```python
from build123d import *

# Parameters (mm, degrees)
F1_DEPTH = 50.8
F2_R     = 2.975
F3_DEPTH = 12
F4_R     = 0.25
F5_DEPTH = 17


with BuildPart() as f1:
    # F0 (on Top) → F1 (new body)
    with BuildSketch(Plane.XY):
        Polygon((-1.9875, 6.35), (-6.35, 6.35), (-6.35, 1.9875), (-2.975, 1.9875), (-2.975, -1.9875), (-6.35, -1.9875), (-6.35, -6.35), (-1.9875, -6.35), (-1.9875, -2.975), (1.9875, -2.975), (1.9875, -6.35), (6.35, -6.35), (6.35, -1.9875), (2.975, -1.9875), (2.975, 1.9875), (6.35, 1.9875), (6.35, 6.35), (1.9875, 6.35), (1.9875, 2.975), (-1.9875, 2.975), align=None)
    extrude(amount=F1_DEPTH)

    # F2 (on face) → F3 (join)
    with BuildSketch(Plane.XY.offset(50.8)):
        Circle(F2_R)
    extrude(amount=F3_DEPTH)

    # F4 (on face) → F5 (cut)
    with BuildSketch(Plane.XY.offset(62.8)):
        with Locations((0, 1.5)):
            Circle(F4_R)
        with Locations((-1.426585, 0.463525)):
            Circle(F4_R)
        with Locations((-0.881678, -1.213525)):
            Circle(F4_R)
        with Locations((0.881678, -1.213525)):
            Circle(F4_R)
        Circle(F4_R)
        with Locations((1.426585, 0.463525)):
            Circle(F4_R)
    extrude(amount=-F5_DEPTH, mode=Mode.SUBTRACT)


solid = f1.part
```
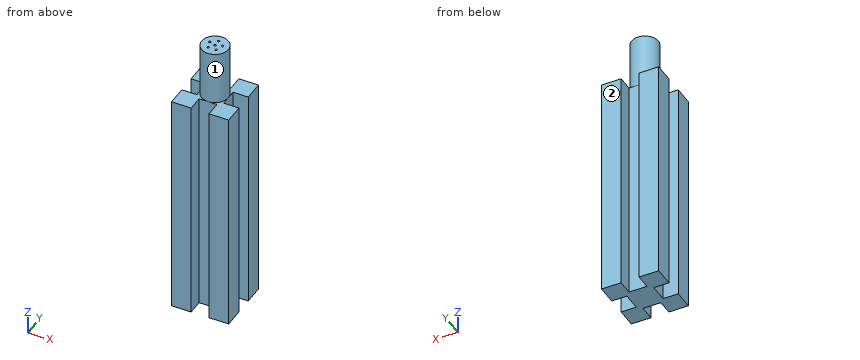
Design review of the part built by this model. Coordinates are the model's own, in mm. Face numbers are marked on the shaded views. A direction names the side the tool comes from. Give positions to 0.01 mm unless a question says otherwise; leave off trailing zeros. Order: outer loops, then holes, each group sorted by start corner. A loop starts at its lowest first (then second) coordinate and runs counter-clockwise, first axis right, second up. Notation, with made-up numbers: M -26.75,3.25 L 7.25,3.25 A27 cw 7.25,30.25 Z; hole C 27.25,-16 d1. An arc over 180 degrees is marked long. One line per question, with ' | ' between items. Start each with the question number.
Q1. Machinability: for the marked faces 1 and 2, which of the approach directions +Z, -Z, +X, -X, +Y, -Y give a long, thin tool a straight path to every point of the face, cutting with its end or side? Answer none if there is none.
Q2. We need section D-D (z = 52.5). Write out the cut boundary in (x, y) (3 decimals).
Q3. For pin 1 Ø1.2 at (x, z) = (0.5, 34) entering from -Y (3 decimals); pin 2 Ø2 at (y, z) = (0, 28.5) entering from +X (3 decimals), all flat-tipped, find the tip position at first contact; note any pin that passes through.
Q4. We need section A-A (y = 3.5). Write out the cut boundary in (x, z), plus the area to 3 significant figures.
Q5. For L1, parallel to Y at x = 0, z = 54.25 (3 decimals); L2, parallel to X at y = 5.75, z = 37, list the stretches that pass through material, from the lowest coordinate up. Write a range as [from, to].
Returned:
1) face 1: +Z | face 2: +Z, -Z, +X, -X, +Y
2) outline: C 0,0 d5.95; hole C -1.427,0.464 d0.5; hole C -0.882,-1.214 d0.5; hole C 0,0 d0.5; hole C 0,1.5 d0.5; hole C 0.882,-1.214 d0.5; hole C 1.427,0.464 d0.5
3) pin 1: y = -2.975 | pin 2: x = 2.975
4) outline: M -6.35,0 L -1.99,0 L -1.99,50.8 L -6.35,50.8 Z; M 1.99,0 L 6.35,0 L 6.35,50.8 L 1.99,50.8 Z | area: 443 mm2
5) L1: [-2.975, -0.25], [0.25, 1.25], [1.75, 2.975] | L2: [-6.35, -1.99], [1.99, 6.35]
